from build123d import *

# Parameters (mm, degrees)
F1_DEPTH = 6.35
F2_R     = 0.762


with BuildPart() as f1:
    # F0 (on Top) → F1 (new body)
    with BuildSketch(Plane.XY):
        with BuildLine():
            Line((-20.574, -2.54), (-16.174591, 0))
            Line((-16.174591, 0), (-20.574, 0))
            ThreePointArc((-20.574, 0), (-22.819064, -0.929936), (-23.749, -3.175))
            Line((-23.749, -3.175), (-23.749, -23.749))
            ThreePointArc((-23.749, -23.749), (-22.819064, -25.994064), (-20.574, -26.924))
            Line((-20.574, -26.924), (21.082, -26.924))
            ThreePointArc((21.082, -26.924), (23.327064, -25.994064), (24.257, -23.749))
            Line((24.257, -23.749), (24.257, -3.175))
            ThreePointArc((24.257, -3.175), (23.327064, -0.929936), (21.082, 0))
            Line((21.082, 0), (16.682591, 0))
            Line((16.682591, 0), (21.082, -2.54))
            Line((21.082, -2.54), (21.082, -23.749))
            Line((21.082, -23.749), (-20.574, -23.749))
            Line((-20.574, -23.749), (-20.574, -2.54))
        make_face()
    extrude(amount=F1_DEPTH)

    # F2
    f2_edges = [f1.edges().sort_by_distance(p)[0] for p in [
        (-20.574, -13.1445, 6.35),
        (-18.374295, -1.27, 6.35),
        (-18.374295, 0, 6.35),
        (-22.819064, -0.929936, 6.35),
        (-23.749, -13.462, 6.35),
        (-22.819064, -25.994064, 6.35),
        (0.254, -26.924, 6.35),
        (23.327064, -25.994064, 6.35),
        (24.257, -13.462, 6.35),
        (23.327064, -0.929936, 6.35),
        (18.882295, 0, 6.35),
        (18.882295, -1.27, 6.35),
        (21.082, -13.1445, 6.35),
        (0.254, -23.749, 6.35),
        (-20.574, -13.1445, 0),
        (-18.374295, -1.27, 0),
        (-18.374295, 0, 0),
        (-22.819064, -0.929936, 0),
        (-23.749, -13.462, 0),
        (-22.819064, -25.994064, 0),
        (0.254, -26.924, 0),
        (23.327064, -25.994064, 0),
        (24.257, -13.462, 0),
        (23.327064, -0.929936, 0),
        (18.882295, 0, 0),
        (18.882295, -1.27, 0),
        (21.082, -13.1445, 0),
        (0.254, -23.749, 0),
    ]]
    fillet(f2_edges, radius=F2_R)


solid = f1.part
The listing builds one solid part. Answer for the finished solid, in the listing's coordinates (mm). A direction names the side the tool comes from. Coordinates: 2 decimals unless noted, no trailing zeros. Order: outer loops, then holes, each group sorted by start corner. A loop starts at its lowest first (then second) coordinate and runs counter-clockwise, first axis right, second up. Notation, with made-up numbers: (55.25, 80) -> (102.25, 80) arc R24 ccw to (102.25, 104) -> close; hole circle Ø7 at (-35, 46). An arc over 180 degrees is marked (long way). Answer in a Markdown table with one row per item. Add a question column.
Item 1: Which of the six approach directions +Z, -Z, +X, -X, +Y, -Y give full straight-line access (tool end or side, diameter ignored) to faces 5 (the face through (23.352, -0.955, 3.141)), 6 (the face through (-18.64, -1.172, 0.229)), 7 (the face through (-18.41, -1.29, 3.14)), 8 (the face through (19.21, -1.21, 6.12))?
Item 2: Find the intervals of material crossed by L1, parallel to X at y = -4.25, z = 3; L2, parallel to Y at x = 18, z = 3; L3, parallel to Y at x = -4, z = 1.5, in increasing order. Write a range as from..to.
Item 3: Find section C-C (z = 2). Write down the section's boundary in (x, y) (3 decimals).
Item 4: Find section A-A (y = -15.25). Write down the section's boundary in (x, z) (3 decimals).
Item 5: Find section B-B (x = 2). Write down the section's boundary in (y, z), then the cut area to 3 significant figures.
Item 6: Determine the mould class of faces 1 (the face through (21.082, -13, 3)), 2 (the face through (24.257, -14, 3)), 3 (the face through (0, -25, 6.35)), 4 (the face through (-18.64, -1.172, 6.121)) for opening direction X: +X half, -X half, draft (parallel to the pull), parting line (faces both ways), or undercut.
Result set:
| question | item | result |
|---|---|---|
| 1 | face 5 | +Z, -Z, +X, +Y |
| 1 | face 6 | -Z |
| 1 | face 7 | +Z, -Z |
| 1 | face 8 | +Z |
| 2 | L1 | x = -23.75..-20.57, 21.08..24.26 |
| 2 | L2 | y = -26.92..-23.75, -0.76..0 |
| 2 | L3 | y = -26.92..-23.75 |
| 3 | outline | (-23.749, -23.749) arc R3.175 ccw to (-20.574, -26.924) -> (21.082, -26.924) arc R3.175 ccw to (24.257, -23.749) -> (24.257, -3.175) arc R3.175 ccw to (21.082, 0) -> (16.683, 0) -> (21.082, -2.54) -> (21.082, -23.749) -> (-20.574, -23.749) -> (-20.574, -2.54) -> (-16.175, 0) -> (-20.574, 0) arc R3.175 ccw to (-23.749, -3.175) -> close |
| 4 | outline | (-23.749, 0.762) arc R0.762 ccw to (-22.987, 0) -> (-21.336, 0) arc R0.762 ccw to (-20.574, 0.762) -> (-20.574, 5.588) arc R0.762 ccw to (-21.336, 6.35) -> (-22.987, 6.35) arc R0.762 ccw to (-23.749, 5.588) -> close; (21.082, 0.762) arc R0.762 ccw to (21.844, 0) -> (23.495, 0) arc R0.762 ccw to (24.257, 0.762) -> (24.257, 5.588) arc R0.762 ccw to (23.495, 6.35) -> (21.844, 6.35) arc R0.762 ccw to (21.082, 5.588) -> close |
| 5 | outline | (-26.92, 0.76) arc R0.76 ccw to (-26.16, 0) -> (-24.51, 0) arc R0.76 ccw to (-23.75, 0.76) -> (-23.75, 5.59) arc R0.76 ccw to (-24.51, 6.35) -> (-26.16, 6.35) arc R0.76 ccw to (-26.92, 5.59) -> close |
| 5 | area | 19.7 mm² |
| 6 | face 1 | undercut |
| 6 | face 2 | +X half |
| 6 | face 3 | draft |
| 6 | face 4 | undercut |
